Design review of the part built by this model. Coordinates are the model's own, in mm. A direction names the side the tool comes from. Coordinates: 2 decimals unless noted, no trailing zeros. Write each loop counter-clockwise with the first axis right and the second up, starting at its lowest first coordinate (ties: lowest second). Pieces come first, ordered by that corner, then holes. Notation, with made-up numbers: (6.5, 28.5) -> (19.5, 28.5) arc R20 ccw to (19.5, 43.5) -> close; hole circle Ø3 at (67.25, -23.75). An arc over 180 degrees is marked (long way). Return JSON: item names as keys, results as strings. Group by question number.
from build123d import *

# Parameters (mm, degrees)
SKETCH_1_R      = 13.25
SKETCH_1_R_2    = 2
SKETCH_1_R_3    = 2.5
SKETCH_1_R_4    = 10
EXTRUDE_1_DEPTH = 5
FILLET_1_R      = 5


with BuildPart() as part:
    # 草图1 → 凸台-拉伸1 (new body)
    with BuildSketch(Plane.XY):
        with BuildLine():
            Line((0, 25), (124.869292101, 25))
            Line((124.869292101, 25), (184, 25))
            ThreePointArc((184, 25), (208.968890762, 1.246793543), (186.490484142, -24.875640469))
            Line((186.490484142, -24.875640469), (124.869292101, -25))
            Line((124.869292101, -25), (0, -25))
            Line((0, -25), (-16, -25))
            Line((-16, -25), (-16, 25))
            Line((-16, 25), (0, 25))
        make_face()
        with Locations((184, 0)):
            Circle(SKETCH_1_R, mode=Mode.SUBTRACT)
        with Locations((5, 16)):
            Circle(SKETCH_1_R_2, mode=Mode.SUBTRACT)
        with Locations(Location((5, -16, 0), (0, 0, 180))):
            Circle(SKETCH_1_R_2, mode=Mode.SUBTRACT)
        with Locations((60, 18)):
            Circle(SKETCH_1_R_3, mode=Mode.SUBTRACT)
        with Locations((124, 18)):
            Circle(SKETCH_1_R_3, mode=Mode.SUBTRACT)
        with Locations((34, 0)):
            Circle(SKETCH_1_R_4, mode=Mode.SUBTRACT)
        with Locations(Location((124, -18, 0), (0, 0, 180))):
            Circle(SKETCH_1_R_3, mode=Mode.SUBTRACT)
        with Locations(Location((60, -18, 0), (0, 0, 180))):
            Circle(SKETCH_1_R_3, mode=Mode.SUBTRACT)
        with Locations((-7, 16)):
            Circle(SKETCH_1_R_2, mode=Mode.SUBTRACT)
        with Locations(Location((-7, -16, 0), (0, 0, 180))):
            Circle(SKETCH_1_R_2, mode=Mode.SUBTRACT)
        with BuildLine():
            Line((75, 12), (110, 12))
            ThreePointArc((110, 12), (113, 9), (110, 6))
            Line((110, 6), (75, 6))
            ThreePointArc((75, 6), (72, 9), (75, 12))
        make_face(mode=Mode.SUBTRACT)
        with BuildLine():
            Line((75, -12), (110, -12))
            ThreePointArc((110, -12), (113, -9), (110, -6))
            Line((110, -6), (75, -6))
            ThreePointArc((75, -6), (72, -9), (75, -12))
        make_face(mode=Mode.SUBTRACT)
        with BuildLine():
            Line((124, 3), (159, 3))
            ThreePointArc((159, 3), (162, 0), (159, -3))
            Line((159, -3), (124, -3))
            ThreePointArc((124, -3), (121, 0), (124, 3))
        make_face(mode=Mode.SUBTRACT)
    extrude(amount=EXTRUDE_1_DEPTH)

    # 圆角1
    fillet_1_edges = [part.edges().sort_by_distance(p)[0] for p in [
        (-16, -25, 2.5),
        (-16, 25, 2.5),
    ]]
    fillet(fillet_1_edges, radius=FILLET_1_R)


solid = part.part
Q1. We need section D-D on x = 60. Write out the cut boundary in (y, z), plus the area to 3 significant figures.
Q2. For faces 4 (the flat face through (92, 12, 2)), 5 (the flat face through (85, 25, 2)), list the 3-axis set-ups (+Z, -Z, +X, -X, +Y, -Y) from which the entire face can be reached by the end or side of a thin tool; tool diameter is ignored.
Q3. For P1, Ø1.5, axis at x = 136.5, z = 3, coming from the -Y side, flat-tipped, find the tip position at first contact; note if it passes through.
Q4. We need section B-B on z = 3.6. State how many separate pieces and enclosed holes the cut face has, plus the area to 3 significant figures.
Q5. We need section A-A on x = 92. Write out the cut boundary in (y, z), plus the area to 3 significant figures.
Q6. We need section C-C on x = 157. Write out the cut boundary in (y, z).
Q7. The part is to be moulded in two halves that separate along Y. For faces 1 (the flat face through (92, -12, 2)), 2 (the cylindrical face through (-14, 24, 3)), 3 (the flat face through (98, 0, 0)), say which applies: +Y half, -Y half, draft (parallel to the pull), parting line (faces both ways), or undercut.
Q8. Wall thickness on L1, parallel to Y at x = 60, z = 1.8; L2, parallel to Y at x = -7, z = 2.3; L3, parallel to Y at x = 148, z = 2.55: over which ranges is each line inside the solid? List them lowest first.
Findings below:
{
 "1": {"outline": "(-25, 0) -> (-20.5, 0) -> (-20.5, 5) -> (-25, 5) -> close; (-15.5, 0) -> (15.5, 0) -> (15.5, 5) -> (-15.5, 5) -> close; (20.5, 0) -> (25, 0) -> (25, 5) -> (20.5, 5) -> close", "area": "200 mm^2"},
 "2": {"face 4": "+Z, -Z", "face 5": "+Z, -Z, +X, -X, +Y"},
 "3": {"P1": "stops at y = -24.98"},
 "4": {"separate pieces": "1", "enclosed holes": "13", "area": "9,260 mm^2"},
 "5": {"outline": "(-25, 0) -> (-12, 0) -> (-12, 5) -> (-25, 5) -> close; (-6, 0) -> (6, 0) -> (6, 5) -> (-6, 5) -> close; (12, 0) -> (25, 0) -> (25, 5) -> (12, 5) -> close", "area": "190 mm^2"},
 "6": {"outline": "(-24.94, 0) -> (-3, 0) -> (-3, 5) -> (-24.94, 5) -> close; (3, 0) -> (25, 0) -> (25, 5) -> (3, 5) -> close"},
 "7": {"face 1": "undercut", "face 2": "+Y half", "face 3": "draft"},
 "8": {"L1": "y = -25 to -20.5, -15.5 to 15.5, 20.5 to 25", "L2": "y = -25 to -18, -14 to 14, 18 to 25", "L3": "y = -24.95 to -3, 3 to 25"}
}
